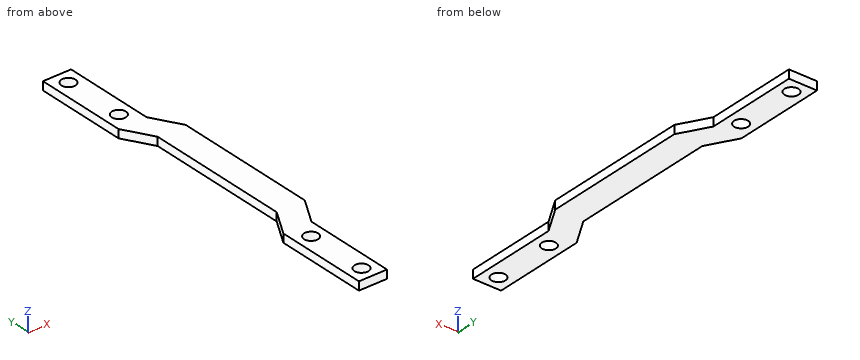
from build123d import *

# Parameters (mm, degrees)
ESQUISSE1_R        = 2.5
BOSS_EXTRU_1_DEPTH = 3


with BuildPart() as part:
    # Esquisse1 → Boss.-Extru.1 (new body)
    with BuildSketch(Plane.XY):
        Polygon((-100.080131723, 30.264285714), (-100.080131723, 63.264285714), (-110.080131723, 63.264285714), (-110.080131723, 30.264285714), (-104.306629031, 20.264285714), (-104.306629031, -31.735714286), (-110.080131723, -41.735714286), (-110.080131723, -74.735714286), (-100.080131723, -74.735714286), (-100.080131723, -41.735714286), (-94.306629031, -31.735714286), (-94.306629031, 20.264285714), align=None)
        with Locations((-105.080131723, 58.264285714)):
            Circle(ESQUISSE1_R, mode=Mode.SUBTRACT)
        with Locations((-105.080131723, 36.264285714)):
            Circle(ESQUISSE1_R, mode=Mode.SUBTRACT)
        with Locations(Location((-105.080131723, -47.735714286, 0), (0, 0, 180))):
            Circle(ESQUISSE1_R, mode=Mode.SUBTRACT)
        with Locations(Location((-105.080131723, -69.735714286, 0), (0, 0, 180))):
            Circle(ESQUISSE1_R, mode=Mode.SUBTRACT)
    extrude(amount=BOSS_EXTRU_1_DEPTH)


solid = part.part
Part model, mm, in its own coordinate system. Coordinates: 2 decimals unless noted, no trailing zeros. Write each loop counter-clockwise with the first axis right and the second up, starting at its lowest first coordinate (ties: lowest second). Pieces come first, ordered by that corner, then holes. Notation, with made-up numbers: (61, 76.5) - (116, 76.5) arc R22 cw to (116, 107.5) - close; hole circle Ø10 at (74.5, 73.5). An arc over 180 degrees is marked (long way). Put each result on its own line as item: value.
1. Probe line 1 along Y through (x, z) = (-105.75, 1); line 2 along X through (y, z) = (-28.5, 0.5); line 3 along X through (y, z) = (-67, 1.05). List the from-to ranges inside material, lowest first. Write a range as [from, to].
Final values:
line 1: y = [-74.74, -72.14], [-67.33, -50.14], [-45.33, -34.24], [22.76, 33.86], [38.67, 55.86], [60.67, 63.26]
line 2: x = [-104.31, -94.31]
line 3: x = [-110.08, -100.08]
2. Band-saw the part on C-C (x = -96). Write the cut outline in (y, z), then the cut area to 3 significant figures.
Final values:
outline: (-34.67, 0) - (23.2, 0) - (23.2, 3) - (-34.67, 3) - close
area: 174 mm²
3. Flat gauge pins, fed straight in: pin 1 Ø0.9 at (y, z) = (-51, 2) entering from +X; pin 2 Ø1.5 at (y, z) = (-13, 1.5) entering from -X. Where does each tip first touch, or does it go through?
Final values:
pin 1: stops at x = -100.08
pin 2: stops at x = -104.31
4. Band-saw the part on A-A (z = 2.45). Write the cut outline in (x, y), then the cut area to 3 significant figures.
Final values:
outline: (-110.08, -74.74) - (-100.08, -74.74) - (-100.08, -41.74) - (-94.31, -31.74) - (-94.31, 20.26) - (-100.08, 30.26) - (-100.08, 63.26) - (-110.08, 63.26) - (-110.08, 30.26) - (-104.31, 20.26) - (-104.31, -31.74) - (-110.08, -41.74) - close; hole circle Ø5 at (-105.08, -69.74); hole circle Ø5 at (-105.08, -47.74); hole circle Ø5 at (-105.08, 36.26); hole circle Ø5 at (-105.08, 58.26)
area: 1,300 mm²
5. Band-saw the part on B-B (y = -7.5). Write the cut outline in (x, z), then the cut area to 3 significant figures.
Final values:
outline: (-104.31, 0) - (-94.31, 0) - (-94.31, 3) - (-104.31, 3) - close
area: 30.0 mm²
